CAD build for the part. Positions are in the model's coordinates, mm. A direction names the side the tool comes from. Give positions to 0.01 mm unless a question says otherwise; leave off trailing zeros. Loops run counter-clockwise (first coordinate to the right, second up) from the corner with the lowest first, then second, coordinate; pieces in that order, holes last. Notation, with made-up numbers: (52, 15) - (87, 15) arc R13 cw to (87, 31) - close; hole circle Ø10 at (-36.75, 45.5). An arc over 180 degrees is marked (long way). Return JSON: item names as keys, results as strings.
from build123d import *

# Parameters (mm, degrees)
SKETCH_1_W               = 100
SKETCH_1_H               = 180
EXTRUDE_1_DEPTH          = 40
SKETCH_2_W               = 79
SKETCH_2_H               = 42
CUT_EXTRUDE_1_DEPTH      = 4
SKETCH_3_W               = 72
SKETCH_3_H               = 40
CUT_EXTRUDE_2_DEPTH      = 27
SKETCH_2_3_R             = 43
CUT_EXTRUDE_3_DEPTH      = 30
CUT_EXTRUDE_4_REACH      = 142.357
CUT_EXTRUDE_4_END_RADIUS = 43
SKETCH_4_R               = 4
SKETCH_5_R               = 2.5
EXTRUDE_2_DEPTH          = 22
CUT_EXTRUDE_5_DEPTH      = 4
CUT_EXTRUDE_6_DEPTH      = 178


with BuildPart() as part:
    # 草图1 → 凸台-拉伸1 (new body)
    with BuildSketch(Plane(origin=(0, 0, 0), x_dir=(1, 0, 0), z_dir=(0, 1, 0))):
        Rectangle(SKETCH_1_W, SKETCH_1_H)
    extrude(amount=EXTRUDE_1_DEPTH)

    # 草图2 → 切除-拉伸1 (cut)
    with BuildSketch(Plane(origin=(0, 40, 0), x_dir=(1, 0, 0), z_dir=(0, 1, 0))):
        with Locations((0, 57)):
            Rectangle(SKETCH_2_W, SKETCH_2_H)
    extrude(amount=-CUT_EXTRUDE_1_DEPTH, mode=Mode.SUBTRACT)

    # 草图3 → 切除-拉伸2 (cut)
    with BuildSketch(Plane(origin=(0, 36, 0), x_dir=(1, 0, 0), z_dir=(0, 1, 0))):
        with Locations((0, 57)):
            Rectangle(SKETCH_3_W, SKETCH_3_H)
    extrude(amount=-CUT_EXTRUDE_2_DEPTH, mode=Mode.SUBTRACT)

    # 草图2<3> → 切除-拉伸3 (cut)
    with BuildSketch(Plane(origin=(0, 40, 0), x_dir=(1, 0, 0), z_dir=(0, 1, 0))):
        with Locations(Location((0, -31, 0), (0, 0, 270))):
            Circle(SKETCH_2_3_R)
    extrude(amount=-CUT_EXTRUDE_3_DEPTH, mode=Mode.SUBTRACT)

    # 切除-拉伸4: up to this cylinder (the profile starts outside it)
    cut_extrude_4_end = Plane(origin=(0, 14, 31), z_dir=(0, 1, 0)) * Cylinder(CUT_EXTRUDE_4_END_RADIUS, 371.714, mode=Mode.PRIVATE)
    # 草图4 → 切除-拉伸4 (cut, up to the surface)
    with BuildSketch(Plane(origin=(50, 0, 0), x_dir=(0, 0, -1), z_dir=(1, 0, 0)), mode=Mode.PRIVATE) as cut_extrude_4_sk1:
        with Locations((-30, 14)):
            Circle(SKETCH_4_R)
    cut_extrude_4_tool1 = extrude(cut_extrude_4_sk1.sketch, amount=-CUT_EXTRUDE_4_REACH, mode=Mode.PRIVATE) - cut_extrude_4_end
    add(cut_extrude_4_tool1.solids().sort_by_distance((50, 14, 30))[0], mode=Mode.SUBTRACT)

    # 草图5 → 凸台-拉伸2 (add)
    with BuildSketch(Plane(origin=(0, 10, 0), x_dir=(1, 0, 0), z_dir=(0, 1, 0))):
        with Locations(Location((-20, -11, 0), (0, 0, 270))):
            Circle(SKETCH_5_R)
        with Locations(Location((20, -11, 0), (0, 0, 90))):
            Circle(SKETCH_5_R)
        with Locations(Location((-20, -51, 0), (0, 0, 90))):
            Circle(SKETCH_5_R)
        with Locations(Location((20, -51, 0), (0, 0, 270))):
            Circle(SKETCH_5_R)
    extrude(amount=EXTRUDE_2_DEPTH)

    # 草图6 → 切除-拉伸5 (cut)
    with BuildSketch(Plane(origin=(0, 40, 0), x_dir=(1, 0, 0), z_dir=(0, 1, 0))):
        with BuildLine():
            Line((-10, 86), (10, 86))
            ThreePointArc((10, 86), (18, 78), (10, 70))
            Line((10, 70), (-10, 70))
            ThreePointArc((-10, 70), (-18, 78), (-10, 86))
        make_face()
        with BuildLine():
            Line((-10, 28), (10, 28))
            ThreePointArc((10, 28), (18, 36), (10, 44))
            Line((10, 44), (-10, 44))
            ThreePointArc((-10, 44), (-18, 36), (-10, 28))
        make_face()
    extrude(amount=-CUT_EXTRUDE_5_DEPTH, mode=Mode.SUBTRACT)

    # 草图8 → 切除-拉伸6 (cut)
    with BuildSketch(Plane(origin=(0, 0, -90), x_dir=(-1, 0, 0), z_dir=(0, 0, -1))):
        Polygon((0, 40), (0, 37), (48.5, 37), (48.5, 38.5), (46.5, 38.5), (46.5, 40), align=None)
        Polygon((-48.5, 37), (0, 37), (0, 40), (-46.5, 40), (-46.5, 38.5), (-48.5, 38.5), align=None)
    extrude(amount=-CUT_EXTRUDE_6_DEPTH, mode=Mode.SUBTRACT)


solid = part.part
1. Cut at A-A, the plane y = 25. Write the cut outline in (x, z).
Values follow:
{"outline": "(-50, -90) - (50, -90) - (50, 90) - (-50, 90) - close; circle Ø5 at (-20, 11); circle Ø5 at (-20, 51); circle Ø5 at (20, 11); circle Ø5 at (20, 51); hole circle Ø86 at (0, 31); hole (-36, -77) - (36, -77) - (36, -37) - (-36, -37) - close"}
2. Drill centre lines: probe 1 along Z at (x, y) = (0, 22.75); probe 2 along Z at (x, y) = (46, 14); probe 3 along Z at (x, y) = (-7, 25). Where is each one in solid material? Low to high.
Values follow:
{"probe 1": "z = -90 to -77, -37 to -12, 74 to 90", "probe 2": "z = -90 to 26, 34 to 90", "probe 3": "z = -90 to -77, -37 to -11.43, 73.43 to 90"}
3. Which spindle directions (+Z, -Z, +X, -X, +Y, -Y) get a long thin tool onto all of the face, cutting with end or side? Do faces 4 (the face through (22.11, 20.85, 52.34)), 5 (the face through (-1, 15, -90)), 6 (the face through (46.405, 17.966, 30.521)). Say none if no direction does.
Values follow:
{"face 4": "+Y", "face 5": "-Z, +X, -X, +Y, -Y", "face 6": "+X"}
4. Pull direction X, two halves, no side cores. Call faces 1 (the face through (15.594, 36.507, -30.281)), 2 (the face through (-1, 0, -1)), 3 (the face through (-50, 20, 1)): +X half, -X half, draft (parallel to the pull), parting line (faces both ways), or undercut.
Values follow:
{"face 1": "undercut", "face 2": "draft", "face 3": "-X half"}
5. Drop flat-ended pins along their axis: P1, Ø2.5, axis at x = 15, y = 38.5, coming from the -Z side; P2, Ø5.5, axis at x = -19, z = 51.5, coming from the +Y side; P3, Ø1.5, axis at x = 32, z = 69.5, coming from the +Y side. Give the stop position or say it passes through.
Values follow:
{"P1": "stops at z = 88", "P2": "stops at y = 32", "P3": "stops at y = 37"}
6. Cut at C-C, the plane y = 34. Write the cut outline in (x, z), plus the area to 3 significant figures.
Values follow:
{"outline": "(-50, -90) - (50, -90) - (50, 90) - (-50, 90) - close; hole circle Ø86 at (0, 31); hole (-36, -77) - (36, -77) - (36, -37) - (-36, -37) - close", "area": "9,310 mm²"}
7. Cut at B-B, the plane y = 14. Write the cut outline in (x, z).
Values follow:
{"outline": "(-50, -90) - (50, -90) - (50, 26) - (42.71, 26) arc R43 cw (long way) to (42.9, 34) - (50, 34) - (50, 90) - (-50, 90) - close; circle Ø5 at (-20, 11); circle Ø5 at (-20, 51); circle Ø5 at (20, 11); circle Ø5 at (20, 51); hole (-36, -77) - (36, -77) - (36, -37) - (-36, -37) - close"}
8. Cut at D-D, the plane z = -30.5. Write the cut outline in (x, y), plus the area to 3 significant figures.
Values follow:
{"outline": "(-50, 0) - (50, 0) - (50, 40) - (46.5, 40) - (46.5, 38.5) - (48.5, 38.5) - (48.5, 37) - (15.81, 37) - (15.81, 36) - (-15.81, 36) - (-15.81, 37) - (-48.5, 37) - (-48.5, 38.5) - (-46.5, 38.5) - (-46.5, 40) - (-50, 40) - close", "area": "3,680 mm²"}
